CAD build for the part. Positions are in the model's coordinates, mm. Face numbers are marked on the shaded views. Give positions to 0.01 mm unless a question says otherwise; leave off trailing zeros. Loops run counter-clockwise (first coordinate to the right, second up) from the corner with the lowest first, then second, coordinate; pieces in that order, holes last. Notation, with made-up numbers: M 80.25,-32.5 L 130.25,-32.5 A21 ccw 130.25,0.5 Z; hole C -14.75,72 d10. An arc over 180 degrees is marked long. Answer as CSV lines item,"result".
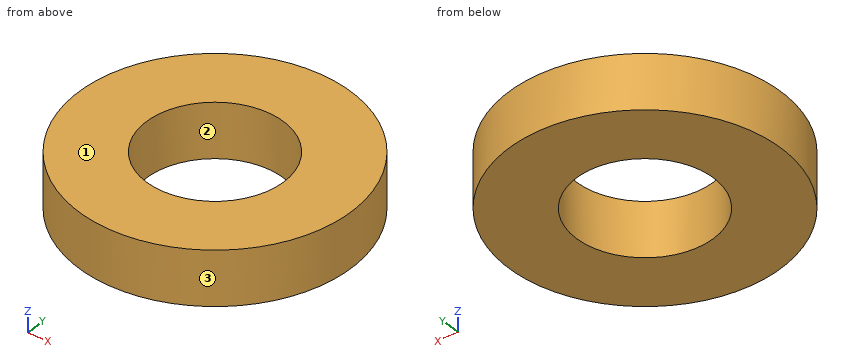
Solid Edge part; units mm, degrees
sketch "Sketch1" plane through (0, 0, 0) normal (0, 0, 1) x (1, 0, 0)
  circle A0 centre (0, 0) radius 6
  circle A1 centre (0, 0) radius 3.2
extrude "Protrusion1" add sketch "Sketch1" along normal blind 1.6
sketch "Sketch2" plane through (0, 0, 1.6) normal (0, 0, 1) x (0, 1, 0)
  circle A0 centre (0, 0) radius 7.9375
extrude "Protrusion2" add sketch "Sketch2" along normal mid plane 3.175
sketch "Sketch3" plane through (0, 0, 3.1875) normal (0, 0, 1) x (1, 0, 0)
  circle A0 centre (0, 0) radius 4
extrude "ExtrudedCutout_1" cut sketch "Sketch3" against normal blind 10.8687
sketch "Sketch4" plane through (0, 0, 0) normal (0, 0, -1) x (0, 1, 0)
  circle A0 centre (0, 0) radius 6
extrude "Cutout1" cut sketch "Sketch4" against normal up to vertex (0.0125 mm away)
properties material "Steel"
1) Band-saw the part on D-D on x = -5. Give the cut face in (y, z), and give its area (3 significant figures).
Answer below:
outline,"M -6.16,0.01 L 6.16,0.01 L 6.16,3.19 L -6.16,3.19 Z"
area,"39.1 mm^2"
2) Mould opens along Y. For the marked faces 1, 2 and 3 say: +Y half, -Y half, draft (parallel to the pull), parting line (faces both ways), or undercut.
Answer below:
face 1,"draft"
face 2,"undercut"
face 3,"parting line"
3) Band-saw the part on C-C on z = 0.95. Give the cut face in (x, y) (1 decimal), and give its area (3 significant figures).
Answer below:
outline,"C 0,0 d15.9; hole C 0,0 d8"
area,"148 mm^2"
4) Flat gauge pin, fed straight in: pin 1 (1.5 mm diameter, centred on y = 4, z = 1, fed in from -X). Where does the tip first touch, or does it go through?
Answer below:
pin 1,"stops at x = -7.24"
5) Band-saw the part on A-A on y = 0. Give the cut face in (x, z), and give its area (3 significant figures).
Answer below:
outline,"M -7.94,0.01 L -4,0.01 L -4,3.19 L -7.94,3.19 Z; M 4,0.01 L 7.94,0.01 L 7.94,3.19 L 4,3.19 Z"
area,"25.0 mm^2"
6) Drill centre lines: line 1 (Y direction, x = 0, z = 2.65); line 2 (X direction, y = 0.75, z = 0.35); line 3 (X direction, y = 2.5, z = 2.8). Where is each one in solid material? Low to high. Write a range as from..to.
Answer below:
line 1,"y = -7.94..-4, 4..7.94"
line 2,"x = -7.9..-3.93, 3.93..7.9"
line 3,"x = -7.53..-3.12, 3.12..7.53"
